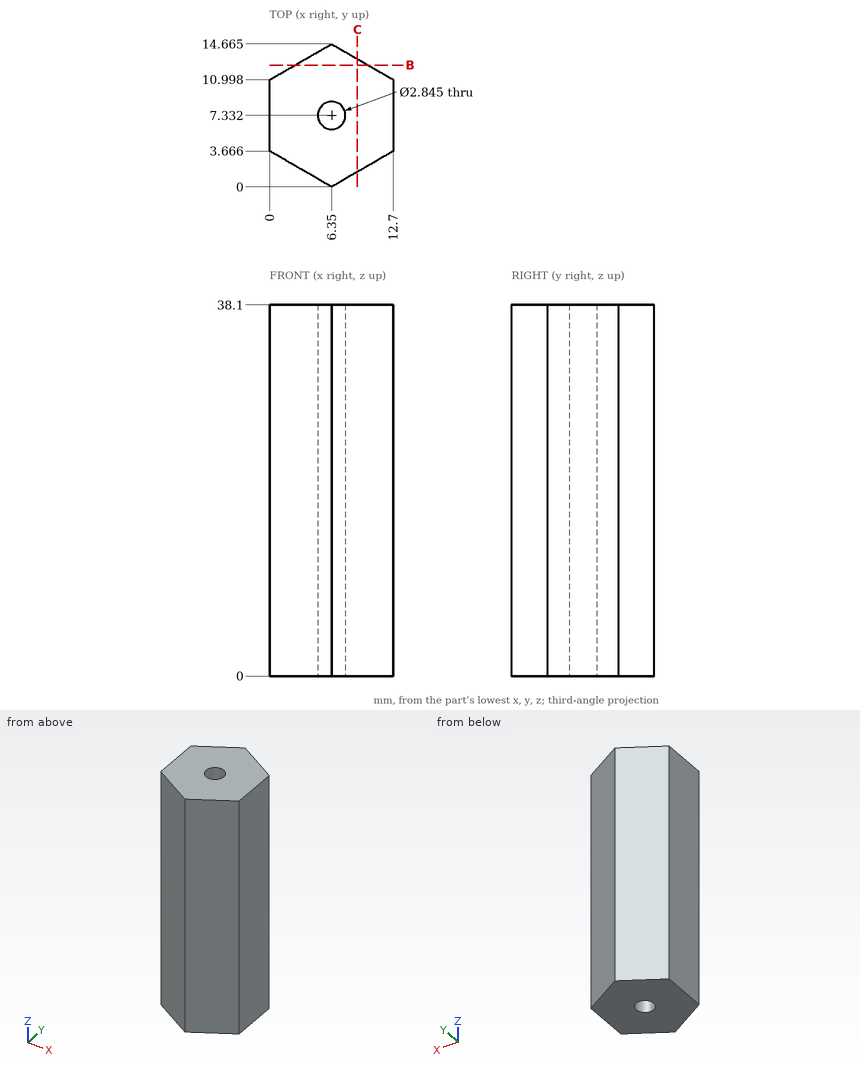
Geometry check sheet. Reference: drawing and pictorial views, mm from the part's lowest x, y, z. Give positions to 0.01 mm unless a question says otherwise; leave off trailing zeros. Order: outer loops, then holes, each group sorted by start corner. A loop starts at its lowest first (then second) coordinate and runs counter-clockwise, first axis right, second up. Notation, with made-up numbers: (80, -7.75) - (119, -7.75) arc R25 cw to (119, 15.25) - close; hole circle Ø8 at (57.25, 17.5). An arc over 180 degrees is marked (long way). Use one line per item in the form item = value.
1) Depth check by flat-ended pin: pin 1 Ø2 at (x, z) = (10, 21) entering from +Y (1 decimal); pin 2 Ø4 at (x, z) = (11, 25) entering from -Y; pin 3 Ø1 at (y, z) = (2.5, 23) entering from +X (1 decimal). Enter the tip coordinate at first touch or a pass-through.
Working result:
pin_1 = 13.1
pin_2 = 1.53
pin_3 = 11.5
2) Material ranges on probe 1 along Y at (x, z) = (7, 2.5) (1 decimal); probe 2 along Y at (x, z) = (7.5, 20) (1 decimal); probe 3 along X at (y, z) = (8.25, 7.5) (1 decimal), recorded low to high. Write a range as from..to.
Working result:
probe_1 = 0.4..6.1, 8.6..14.3
probe_2 = 0.7..6.5, 8.2..14
probe_3 = 0..5.3, 7.4..12.7
3) Sectioned sample at B-B (y = 12.5). Record the boundary of the cut face in (x, z), and give its area (3 significant figures).
Working result:
outline = (2.6, 0) - (10.1, 0) - (10.1, 38.1) - (2.6, 38.1) - close
area = 286 mm^2
4) Sectioned sample at C-C (x = 9). Record the boundary of the cut face in (y, z) (1 decimal).
Working result:
outline = (1.5, 0) - (13.1, 0) - (13.1, 38.1) - (1.5, 38.1) - close
